Read the model definition and answer for the solid it produces. Units are mm, in the model's axes. A direction names the side the tool comes from. Give positions to 0.01 mm unless a question says otherwise; leave off trailing zeros. Write each loop counter-clockwise with the first axis right and the second up, starting at its lowest first coordinate (ties: lowest second). Pieces come first, ordered by that corner, then holes. Notation, with made-up numbers: M 53.5,68.5 L 100.5,68.5 A18 cw 100.5,95.5 Z; hole C 79,21.5 d9. An arc over 180 degrees is marked long. Answer as CSV lines item,"result". Start each with the question number.
```python
from build123d import *

# Parameters (mm, degrees)
SKETCH1_R           = 23.276074499
SKETCH1_R_2         = 2.0193
BOSS_EXTRUDE1_DEPTH = 6
SKETCH2_R           = 17.46
SKETCH2_R_2         = 15
BOSS_EXTRUDE2_DEPTH = 2
CUT_EXTRUDE2_START  = -1.8125
SKETCH4_R           = 15
CUT_EXTRUDE2_DEPTH  = 1.8125
CHAMFER4_SIZE       = 2.5
CHAMFER5_SIZE       = 1
CUT_EXTRUDE3_DEPTH  = 20.5


with BuildPart() as part:
    # Sketch1 → Boss-Extrude1 (new body)
    with BuildSketch(Plane(origin=(0, 0, 0), x_dir=(0, 0, -1), z_dir=(1, 0, 0))):
        Circle(SKETCH1_R)
        with Locations((0, 20.64)):
            Circle(SKETCH1_R_2, mode=Mode.SUBTRACT)
        with Locations((17.874764334, 10.32)):
            Circle(SKETCH1_R_2, mode=Mode.SUBTRACT)
        with Locations((17.874764334, -10.32)):
            Circle(SKETCH1_R_2, mode=Mode.SUBTRACT)
        with Locations((0, -20.64)):
            Circle(SKETCH1_R_2, mode=Mode.SUBTRACT)
        with Locations((-17.874764334, -10.32)):
            Circle(SKETCH1_R_2, mode=Mode.SUBTRACT)
        with Locations((-17.874764334, 10.32)):
            Circle(SKETCH1_R_2, mode=Mode.SUBTRACT)
    extrude(amount=BOSS_EXTRUDE1_DEPTH)

    # Sketch2 → Boss-Extrude2 (add)
    with BuildSketch(Plane.ZY):
        with Locations(Location((0, 0, 0), (0, 0, 180))):
            Circle(SKETCH2_R)
        Circle(SKETCH2_R_2, mode=Mode.SUBTRACT)
    extrude(amount=BOSS_EXTRUDE2_DEPTH)

    # Sketch4 → Cut-Extrude2 (cut)
    with BuildSketch(Plane.ZY.offset(CUT_EXTRUDE2_START)):
        Circle(SKETCH4_R)
    extrude(amount=CUT_EXTRUDE2_DEPTH, mode=Mode.SUBTRACT)

    # Chamfer4
    chamfer4_edges = [part.edges().sort_by_distance(p)[0] for p in [
        (1.8125, 0, -15),
    ]]
    chamfer(chamfer4_edges, length=CHAMFER4_SIZE)

    # Chamfer5
    chamfer5_edges = [part.edges().sort_by_distance(p)[0] for p in [
        (-2, 0, 17.46),
    ]]
    chamfer(chamfer5_edges, length=CHAMFER5_SIZE)

    # Sketch7 → Cut-Extrude3 (cut)
    with BuildSketch(Plane(origin=(6, 0, 0), x_dir=(0, 0, -1), z_dir=(1, 0, 0))):
        with BuildLine():
            Line((-2.5, 3.122498999), (-2.5, 5.422498999))
            Line((-2.5, 5.422498999), (2.5, 5.422498999))
            Line((2.5, 5.422498999), (2.5, 3.122498999))
            ThreePointArc((2.5, 3.122498999), (0, -4), (-2.5, 3.122498999))
        make_face()
    extrude(amount=-CUT_EXTRUDE3_DEPTH, mode=Mode.SUBTRACT)


solid = part.part
```
1. Find section D-D on y = 10.32. State how many separate pieces and enclosed holes the cut face has, then the cut area to 3 significant figures.
2. Find the intervals of material crossed by line 1 (Y direction, x = 2.6, z = 0); line 2 (Y direction, x = 4.25, z = 17); line 3 (X direction, y = -17, z = 11.5), in increasing order. Write a range as [from, to].
3. For faces 4 (the face through (6, -5, 0)), 5 (the face through (4, 5.422, 0)), 6 (the face through (1.812, 3, -3)), determine the directions among +Z, -Z, +X, -X, +Y, -Y from which every point of the face is accessible in a straight line to the end or side of a thin tool.
4. Find section A-A on y = 0. Determine the outline of the cut face in (x, z).
5. Find section B-B on x = 3. Determine the outline of the cut face in (y, z), then the cut area to 3 significant figures.
6. Given pin 1 (2 mm diameter, centred on x = 1.5, z = 10.5, fed in from -Y); pin 2 (10.5 mm diameter, centred on y = 0, z = 0, fed in from -X); pin 3 (2 mm diameter, centred on x = 3.5, z = 0, fed in from -Y); pin 4 (5.5 mm diameter, centred on y = -20.64, z = 0, fed in from +X), each flat-ended and moving along its own axis, determine where each tip first touches the part or whether it passes through.
7. Find section C-C on y = 20. Determine the outline of the cut face in (x, z), then the cut area to 3 significant figures.
8. Determine the mould class of faces 1 (the face through (2.958, 10.409, -15.857)), 2 (the face through (-2, -4, -15)), 3 (the face through (-0.49, -17.31, 2.27)) for opening direction Y: +Y half, -Y half, draft (parallel to the pull), parting line (faces both ways), or undercut.
Computed:
1,separate pieces,"3"
1,enclosed holes,"0"
1,area,"183 mm^2"
2,line 1,"y = [-23.28, -22.66], [-18.62, -4], [5.42, 18.62], [22.66, 23.28]"
2,line 2,"y = [-15.9, -12.14], [-8.5, 8.5], [12.14, 15.9]"
2,line 3,"x = [0, 6]"
3,face 4,"+Z, -Z, +X, +Y, -Y"
3,face 5,"+X, -X"
3,face 6,"-X"
4,outline,"M -2,-16.46 L -1,-17.46 L 0,-17.46 L 0,-23.28 L 6,-23.28 L 6,-4 L 1.81,-4 L 1.81,-12.5 L -0.69,-15 L -2,-15 Z; M -2,15 L -0.69,15 L 1.81,12.5 L 1.81,4 L 6,4 L 6,23.28 L 0,23.28 L 0,17.46 L -1,17.46 L -2,16.46 Z"
5,outline,"C 0,0 d46.55; hole C -20.64,0 d4.04; hole C -10.32,-17.87 d4.04; hole C -10.32,17.87 d4.04; hole M 3.12,-2.5 L 5.42,-2.5 L 5.42,2.5 L 3.12,2.5 A4 ccw long Z; hole C 10.32,-17.87 d4.04; hole C 10.32,17.87 d4.04; hole C 20.64,0 d4.04"
5,area,"1,570 mm^2"
6,pin 1,"stops at y = -21.25"
6,pin 2,"stops at x = 1.81"
6,pin 3,"stops at y = -23.28"
6,pin 4,"stops at x = 6"
7,outline,"M 0,-11.91 L 6,-11.91 L 6,-1.92 L 0,-1.92 Z; M 0,1.92 L 6,1.92 L 6,11.91 L 0,11.91 Z"
7,area,"120 mm^2"
8,face 1,"undercut"
8,face 2,"draft"
8,face 3,"parting line"
